```python
from build123d import *

# Parameters (mm, degrees)
SKETCH1_R           = 4
BOSS_EXTRUDE1_DEPTH = 2


with BuildPart() as part:
    # Sketch1 → Boss-Extrude1 (new body)
    with BuildSketch(Plane.XY):
        with BuildLine():
            Line((-75, 0), (-75, -20))
            Line((-75, -20), (75, -20))
            Line((75, -20), (75, 0))
            ThreePointArc((75, 0), (0, 75), (-75, 0))
        make_face()
        with Locations((-65, 0)):
            Circle(SKETCH1_R, mode=Mode.SUBTRACT)
        Circle(SKETCH1_R, mode=Mode.SUBTRACT)
        with Locations((-63.579594048, 13.514259903)):
            Circle(SKETCH1_R, mode=Mode.SUBTRACT)
        with Locations((-59.380454747, 26.4378818)):
            Circle(SKETCH1_R, mode=Mode.SUBTRACT)
        with Locations((-52.586104634, 38.206041399)):
            Circle(SKETCH1_R, mode=Mode.SUBTRACT)
        with Locations((-43.493489413, 48.304413656)):
            Circle(SKETCH1_R, mode=Mode.SUBTRACT)
        with Locations((-32.5, 56.291651246)):
            Circle(SKETCH1_R, mode=Mode.SUBTRACT)
        with Locations((-20.086104634, 61.818673559)):
            Circle(SKETCH1_R, mode=Mode.SUBTRACT)
        with Locations((-6.794350112, 64.643923199)):
            Circle(SKETCH1_R, mode=Mode.SUBTRACT)
        with Locations((6.794350112, 64.643923199)):
            Circle(SKETCH1_R, mode=Mode.SUBTRACT)
        with Locations((20.086104634, 61.818673559)):
            Circle(SKETCH1_R, mode=Mode.SUBTRACT)
        with Locations((32.5, 56.291651246)):
            Circle(SKETCH1_R, mode=Mode.SUBTRACT)
        with Locations((43.493489413, 48.304413656)):
            Circle(SKETCH1_R, mode=Mode.SUBTRACT)
        with Locations((52.586104634, 38.206041399)):
            Circle(SKETCH1_R, mode=Mode.SUBTRACT)
        with Locations((59.380454747, 26.4378818)):
            Circle(SKETCH1_R, mode=Mode.SUBTRACT)
        with Locations((63.579594048, 13.514259903)):
            Circle(SKETCH1_R, mode=Mode.SUBTRACT)
        with Locations((65, 0)):
            Circle(SKETCH1_R, mode=Mode.SUBTRACT)
    extrude(amount=BOSS_EXTRUDE1_DEPTH)


solid = part.part
```
Part model, mm, in its own coordinate system. Round coordinates to 2 decimals unless told otherwise and drop trailing zeros. Order: outer loops, then holes, each group sorted by start corner. A loop starts at its lowest first (then second) coordinate and runs counter-clockwise, first axis right, second up. Notation, with made-up numbers: M -10.5,-37 L 29.5,-37 A19 cw 29.5,-25 Z; hole C 74.25,-36.75 d2. An arc over 180 degrees is marked long. Put each result on its own line as item: value. Start each with the question number.
1. Two-plate mould, pull along X, no slides. Class faces 1 (the face through (40.55, 51.01, 0.99)), 2 (the face through (1.65, 74.98, 0.99)), 3 (the face through (-1, 18, 2)): +X half, -X half, draft (parallel to the pull), parting line (faces both ways), or undercut.
2. Slice it at A-A on x = -21.5. List the corners of the cut face in (y, z), then the cut area to 3 significant figures.
3. Drop a flat-ended pin along its axis: pin 1 (7 mm diameter, centred on x = 63.58, y = 13.51, fed in from +Z). Give the stop position or say it passes through.
4. Slice it at C-C on z = 0.6. State how many separate pieces and enclosed holes the cut face has, then the cut area to 3 significant figures.
5. Drill centre lines: probe 1 along Y at (x, z) = (32.5, 0.7); probe 2 along Y at (x, z) = (61.5, 1.3); probe 3 along Y at (x, z) = (0, 0.85). Where is each one in solid material? Low to high. Write a range as [from, to].
6. Slice it at B-B on x = 65. List the corners of the cut face in (y, z).
7. Slice it at D-D on x = 26.5. List the corners of the cut face in (y, z), then the cut area to 3 significant figures.
Findings:
1. face 1: undercut
1. face 2: parting line
1. face 3: draft
2. outline: M -20,0 L 58.08,0 L 58.08,2 L -20,2 Z; M 65.56,0 L 71.85,0 L 71.85,2 L 65.56,2 Z
2. area: 169 mm2
3. pin 1: through
4. separate pieces: 1
4. enclosed holes: 17
4. area: 11,000 mm2
5. probe 1: [-20, 52.29], [60.29, 67.59]
5. probe 2: [-20, -1.94], [1.94, 10.1], [16.93, 23.05], [29.83, 42.93]
5. probe 3: [-20, -4], [4, 75]
6. outline: M -20,0 L -4,0 L -4,2 L -20,2 Z; M 4,0 L 9.77,0 L 9.77,2 L 4,2 Z; M 17.25,0 L 37.42,0 L 37.42,2 L 17.25,2 Z
7. outline: M -20,0 L 70.16,0 L 70.16,2 L -20,2 Z
7. area: 180 mm2
